```python
from build123d import *

# Parameters (mm, degrees)
BOSS_EXTRUDE1_DEPTH = 20
SKETCH2_W           = 4
SKETCH2_H           = 20
BOSS_EXTRUDE2_DEPTH = 20
SKETCH3_W           = 46
SKETCH3_H           = 12
CUT_EXTRUDE1_DEPTH  = 46
SKETCH4_R           = 11
CUT_EXTRUDE2_DEPTH  = 8
FILLET1_R           = 10


with BuildPart() as part:
    # Sketch1 → Boss-Extrude1 (new body)
    with BuildSketch(Plane(origin=(0, 0, 0), x_dir=(1, 0, 0), z_dir=(0, 1, 0))):
        Polygon((-50, 50), (0, 0), (0, 140), (-50, 140), align=None)
    extrude(amount=BOSS_EXTRUDE1_DEPTH)

    # Sketch2 → Boss-Extrude2 (add)
    with BuildSketch(Plane(origin=(0, 0, 0), x_dir=(0, 0, -1), z_dir=(1, 0, 0))):
        with Locations((42, 10)):
            Rectangle(SKETCH2_W, SKETCH2_H)
    extrude(amount=BOSS_EXTRUDE2_DEPTH)

    # Sketch3 → Cut-Extrude1 (cut)
    with BuildSketch(Plane.ZY.offset(50)):
        with Locations((-23, 10)):
            Rectangle(SKETCH3_W, SKETCH3_H)
    extrude(amount=-CUT_EXTRUDE1_DEPTH, mode=Mode.SUBTRACT)

    # Sketch4 → Cut-Extrude2 (cut)
    with BuildSketch(Plane.XZ):
        with Locations((-25, -54)):
            Circle(SKETCH4_R)
        with Locations((-25, -114)):
            Circle(SKETCH4_R)
    extrude(amount=-CUT_EXTRUDE2_DEPTH, mode=Mode.SUBTRACT)

    # Fillet1
    fillet1_edges = [part.edges().sort_by_distance(p)[0] for p in [
        (0, 10, -44),
    ]]
    fillet(fillet1_edges, radius=FILLET1_R)


solid = part.part
```
Geometry check sheet. Reference: the model listing, model coordinates, mm. A direction names the side the tool comes from. Coordinates: 2 decimals unless noted, no trailing zeros. Order: outer loops, then holes, each group sorted by start corner. A loop starts at its lowest first (then second) coordinate and runs counter-clockwise, first axis right, second up.
Item 1: Tool access check on faces 5 (the cylindrical face through (-27.38, 3.94, -64.74)), 6 (the flat face through (-16, 4, -35)), 7 (the flat face through (10, 10, -40)), 8 (the flat face through (-23, 20, -87)). Record the directions out of +Z, -Z, +X, -X, +Y, -Y that give a thin tool (end or side, any length) a straight path to the whole face; none if there is none.
Item 2: Section check A-A (x = -25). Enter the section's corners in (y, z), plus the area to 3 significant figures.
Item 3: Scan lines: line 1 along X through (y, z) = (4.75, -54); line 2 along Y through (x, z) = (-13, -45); line 3 along Z through (x, y) = (-25, 4.25). Record each from-to range of solid material in increasing order.
Item 4: Section check C-C (z = -24.5). Enter the section's corners in (x, y).
Item 5: Mould release check, pull along X, two halves, no side actions. Record for faces 1 (the flat face through (-25, 8, -114)), 2 (the flat face through (-4, 10, -25)), 3 (the flat face through (15, 10, -44)), 4 (the flat face through (0, 10, -96)): released by +X, released by -X, zero draft, split by the parting line, or undercut.
Item 6: Section check B-B (y = 10.25). Enter the section's corners in (x, z), plus the area to 3 significant figures.
Item 7: Depth check by flat-ended pin: pin 1 (5 mm diameter, centred on x = 11, y = 16, fed in from +Z); pin 2 (1.5 mm diameter, centred on y = 5.5, z = -86, fed in from +X); pin 3 (20 mm diameter, centred on x = -25, z = -114, fed in from -Y). Enter the tip coordinate at first touch or a pass-through.
Item 8: Section check D-D (y = 18). Enter the section's corners in (x, z).
Check sheet entries:
1. face 5: -Y
1. face 6: +Z, -X
1. face 7: +Z, +X, +Y, -Y
1. face 8: +Z, -Z, +X, -X, +Y
2. outline: (0, -140) - (20, -140) - (20, -25) - (16, -25) - (16, -46) - (8, -46) - (8, -65) - (0, -65) - (0, -103) - (8, -103) - (8, -125) - (0, -125) - close; (0, -43) - (4, -43) - (4, -25) - (0, -25) - close
2. area: 1,710 mm2
3. line 1: x = -50 to -36, -14 to 0
3. line 2: y = 0 to 4, 16 to 20
3. line 3: z = -140 to -125, -103 to -65
4. outline: (-24.5, 0) - (0, 0) - (0, 20) - (-24.5, 20) - (-24.5, 16) - (-4, 16) - (-4, 4) - (-24.5, 4) - close
5. face 1: undercut
5. face 2: released by -X
5. face 3: zero draft
5. face 4: released by +X
6. outline: (-50, -140) - (0, -140) - (0, -54) arc R10 cw to (10, -44) - (20, -44) - (20, -40) - (0, -40) - (0, 0) - (-4, -4) - (-4, -46) - (-46, -46) - (-50, -50) - close
6. area: 4,970 mm2
7. pin 1: stops at z = -40
7. pin 2: stops at x = 0
7. pin 3: stops at y = 8
8. outline: (-50, -140) - (0, -140) - (0, -54) arc R10 cw to (10, -44) - (20, -44) - (20, -40) - (0, -40) - (0, 0) - (-50, -50) - close
